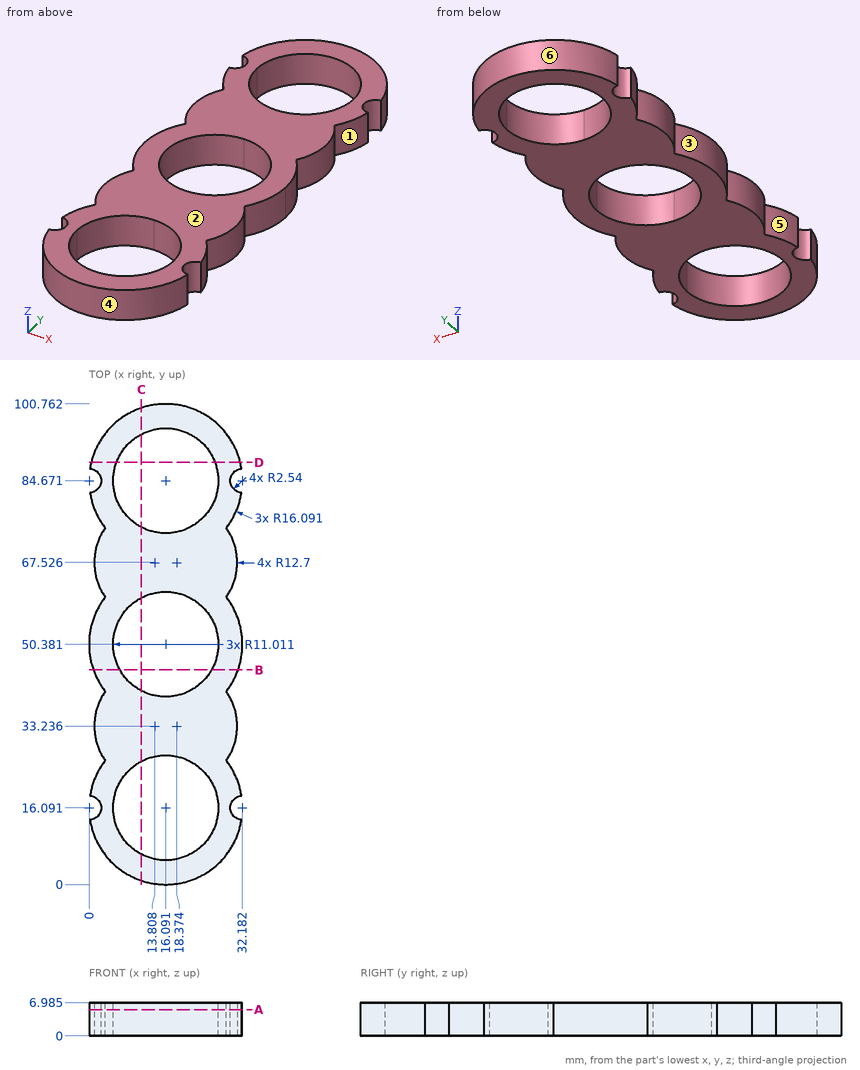
Job drawing, mm, ordinate dimensions from the low corner. One solid piece. A direction names the side the tool comes from. Round coordinates to 2 decimals unless told otherwise and drop trailing zeros. Write each loop counter-clockwise with the first axis right and the second up, starting at its lowest first coordinate (ties: lowest second). Pieces come first, ordered by that corner, then holes. Notation, with made-up numbers: M 53.25,1 L 84.25,1 A10 cw 84.25,7 Z; hole C 62,36.5 d6. An arc over 180 degrees is marked long. Return JSON: item names as keys, results as strings. Group by question number.
(1) Saw through at B-B on y = 45. Write the cut outline in (x, z) (1 decimal).
(2) Two-plate mould, pull along Y, no slides. Class the marked faces 3, 4, 5 and 6: +Y half, -Y half, draft (parallel to the pull), parting line (faces both ways), or undercut.
(3) Drill centre lines: probe 1 along Y at (x, z) = (10.5, 4) (1 decimal); probe 2 along Y at (x, z) = (9, 1) (1 decimal); probe 3 along X at (y, z) = (16, 0.5). Where is each one in solid material? Low to high.
(4) Saw through at D-D on y = 88.5. Write the cut outline in (x, z) (1 decimal).
(5) Saw through at A-A on z = 5.5. Write the cut outline in (x, y).
(6) Saw through at C-C on x = 11. Write the cut outline in (y, z) (1 decimal), then the cut area to 3 significant figures.
(7) Which spindle directions (+Z, -Z, +X, -X, +Y, -Y) get a long thin tool onto all of the face, cutting with end or side? Do the marked faces 1 and 2. Say none if no direction does.
(8) Pin check, flat tips, straight feed: pin 1 Ø1 at (x, y) = (16.5, 75.5) entering from -Z; pin 2 Ø3 at (x, z) = (18, 2) entering from +Y; pin 3 Ø1 at (x, z) = (21, 1) entering from +Y; pin 4 Ø1 at (x, z) = (6.5, 1) entering from -Y (1 decimal). Stop position of each tip, or through.
Returned:
{
 "1": {"outline": "M 0.9,0 L 6.5,0 L 6.5,7 L 0.9,7 Z; M 25.7,0 L 31.3,0 L 31.3,7 L 25.7,7 Z"},
 "2": {"face 3": "undercut", "face 4": "-Y half", "face 5": "undercut", "face 6": "+Y half"},
 "3": {"probe 1": "1 to 6.6, 25.6 to 40.9, 59.9 to 75.2, 94.2 to 99.8", "probe 2": "1.6 to 7.7, 24.5 to 42, 58.8 to 76.2, 93.1 to 99.1", "probe 3": "2.54 to 5.08, 27.1 to 29.64"},
 "4": {"outline": "M 0.5,0 L 5.8,0 L 5.8,7 L 0.5,7 Z; M 26.4,0 L 31.7,0 L 31.7,7 L 26.4,7 Z"},
 "5": {"outline": "M 0.2,13.56 A16.09 ccw 31.98,13.56 A2.54 cw 31.98,18.62 A16.09 ccw 28.79,25.97 A12.7 ccw 28.79,40.5 A16.09 ccw 28.79,60.26 A12.7 ccw 28.79,74.79 A16.09 ccw 31.98,82.14 A2.54 cw 31.98,87.2 A16.09 ccw 0.2,87.2 A2.54 cw 0.2,82.14 A16.09 ccw 3.39,74.79 A12.7 ccw 3.39,60.26 A16.09 ccw 3.39,40.5 A12.7 ccw 3.39,25.97 A16.09 ccw 0.2,18.62 A2.54 cw Z; hole C 16.09,16.09 d22.02; hole C 16.09,50.38 d22.02; hole C 16.09,84.67 d22.02"},
 "6": {"outline": "M 0.8,0 L 6.3,0 L 6.3,7 L 0.8,7 Z; M 25.9,0 L 40.6,0 L 40.6,7 L 25.9,7 Z; M 60.1,0 L 74.9,0 L 74.9,7 L 60.1,7 Z; M 94.4,0 L 99.9,0 L 99.9,7 L 94.4,7 Z", "area": "283 mm²"},
 "7": {"face 1": "+Z, -Z, +X", "face 2": "+Z, +X, -X, +Y, -Y"},
 "8": {"pin 1": "through", "pin 2": "y = 100.76", "pin 3": "y = 100.15", "pin 4": "y = 2.8"}
}
